Read the model definition and answer for the solid it produces. Units are mm, in the model's axes. Face numbers are marked on the shaded views. A direction names the side the tool comes from. Round coordinates to 2 decimals unless told otherwise and drop trailing zeros. Write each loop counter-clockwise with the first axis right and the second up, starting at its lowest first coordinate (ties: lowest second). Pieces come first, ordered by that corner, then holes. Notation, with made-up numbers: (8, 88) - (64, 88) arc R27 ccw to (64, 107) - close; hole circle Ø3 at (-29.75, -5). An arc over 180 degrees is marked (long way). Use one line per item in the form item = value. Start each with the question number.
1) Each of these flat-tipped pins is pushed along its axis until it touches: pin 1 (1.6 mm diameter, centred on x = 20.5, z = -1, fed in from +Y); pin 2 (3 mm diameter, centred on x = 15.41, z = -16.25, fed in from -Y); pin 3 (1.1 mm diameter, centred on x = 9, y = 3.5, fed in from -Z). Where does it stop, or does it pass through?
2) The part is cut by section B-B, the plane x = 21.75. Give the vertices of the cut face in (y, z), plus the area to 3 significant figures.
3) The part is cut by section C-C, the plane z = -6.25. Give the vertices of the cut face in (x, y), plus the area to 3 significant figures.
4) For the marked faces 1, 2 and 3, determine the directions among +Z, -Z, +X, -X, +Y, -Y from which every point of the face is accessible in a straight line to the end or side of a thin tool.
5) Consider line 1 along X through (y, z) = (2.3, -11.25); line 2 along Z through (x, y) = (16, 1.6); line 3 along Z through (x, y) = (16, 3.85). Determine where each line is inside the solid, lowest interval first. Write a range as from..to.
6) The part is cut by section D-D, the plane z = -9.5. Give the vertices of the cut face in (x, y), plus the area to 3 significant figures.
7) The part is cut by section A-A, the plane y = 3.35. Give the vertices of the cut face in (x, z).
from build123d import *

# Parameters (mm, degrees)
SKETCH_1_R          = 1.05
EXTRUDE_1_DEPTH     = 2
EXTRUDE_START       = 2
SKETCH_1_3_R        = 1.05
EXTRUDE_2_DEPTH     = 2.25
CUT_EXTRUDE_1_DEPTH = 2
SKETCH_3_R          = 1.15
CUT_EXTRUDE_2_DEPTH = 5.25
CHAMFER_1_SIZE      = 1.2


with BuildPart() as part:
    # Эскиз1 → Бобышка-Вытянуть1 (new body)
    with BuildSketch(Plane(origin=(0, 0, 0), x_dir=(1, 0, 0), z_dir=(0, 1, 0))):
        with BuildLine():
            Line((0.878934798, 22.5), (0.878934798, 20.5))
            ThreePointArc((0.878934798, 20.5), (2.615780546, 11.25), (0.878934798, 2))
            Line((0.878934798, 2), (0.878934798, 0))
            Line((0.878934798, 0), (27, 0))
            ThreePointArc((27, 0), (29.615780546, 11.25), (27, 22.5))
            Line((27, 22.5), (0.878934798, 22.5))
        make_face()
        with Locations((16, 11.25)):
            Circle(SKETCH_1_R, mode=Mode.SUBTRACT)
    extrude(amount=EXTRUDE_1_DEPTH)

    # Эскиз1<3> → Бобышка-Вытянуть2 (add)
    with BuildSketch(Plane(origin=(0, 0, 0), x_dir=(1, 0, 0), z_dir=(0, 1, 0)).offset(EXTRUDE_START)):
        with BuildLine():
            Line((27.878934798, 20.5), (0.878934798, 20.5))
            ThreePointArc((0.878934798, 20.5), (2.615780546, 11.25), (0.878934798, 2))
            Line((0.878934798, 2), (27.878934798, 2))
            ThreePointArc((27.878934798, 2), (29.615780546, 11.25), (27.878934798, 20.5))
        make_face()
        with Locations((16, 11.25)):
            Circle(SKETCH_1_3_R, mode=Mode.SUBTRACT)
    extrude(amount=EXTRUDE_2_DEPTH)

    # Эскиз2 → Вырез-Вытянуть1 (cut)
    with BuildSketch(Plane.XZ):
        with BuildLine():
            Line((6.079834852, 0), (0.878934798, 0))
            Line((0.878934798, 0), (0.878934798, -22.5))
            Line((0.878934798, -22.5), (6.079834852, -22.5))
            ThreePointArc((6.079834852, -22.5), (2.615780546, -11.25), (6.079834852, 0))
        make_face()
    extrude(amount=-CUT_EXTRUDE_1_DEPTH, mode=Mode.SUBTRACT)

    # Эскиз3 → Вырез-Вытянуть2 (cut, through all)
    with BuildSketch(Plane(origin=(0, 4.25, 0), x_dir=(1, 0, 0), z_dir=(0, 1, 0))):
        with Locations((15.410523666, 6.25)):
            Circle(SKETCH_3_R)
        with Locations((15.410523666, 16.25)):
            Circle(SKETCH_3_R)
    extrude(amount=-CUT_EXTRUDE_2_DEPTH, mode=Mode.SUBTRACT)

    # Фаска1
    chamfer_1_edges = [part.edges().sort_by_distance(p)[0] for p in [
        (14.260523666, 0, -16.25),
        (14.260523666, 0, -6.25),
    ]]
    chamfer(chamfer_1_edges, length=CHAMFER_1_SIZE)


solid = part.part
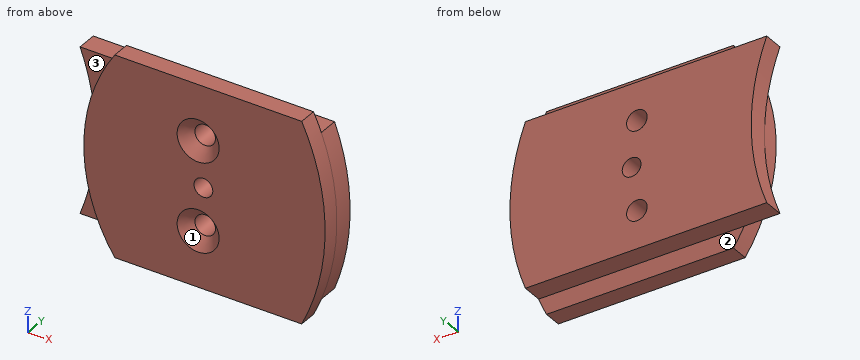
Geometry results:
q1.pin_1 = 2
q1.pin_2 = 0.85
q1.pin_3 = -20.5
q2.outline = (0, -22.5) - (2, -22.5) - (2, -20.5) - (4.25, -20.5) - (4.25, -2) - (2, -2) - (2, 0) - (0, 0) - close
q2.area = 86.6 mm2
q3.outline = (2.12, 2) - (3.25, 2) - (3.25, 0) - (13.06, 0) - (14.26, 1.2) - (14.26, 4.25) - (2.12, 4.25) - close; (16.56, 1.2) - (17.76, 0) - (29.12, 0) - (29.12, 4.25) - (16.56, 4.25) - close
q3.area = 101 mm2
q4.face_1 = -Y
q4.face_2 = -Z, +X, -X, +Y
q4.face_3 = +Z, -X, -Y
q5.line_1 = 2.62..14.95, 17.05..29.62
q5.line_2 = -22.5..-17.24, -15.26..-12.3, -10.2..-7.24, -5.26..0
q5.line_3 = -20.5..-17.24, -15.26..-12.3, -10.2..-7.24, -5.26..-2
q6.outline = (2.56, 2) - (2.69, 2) - (2.69, 0) - (29.56, 0) - (29.56, 4.25) - (2.56, 4.25) - close
q6.area = 114 mm2
q7.outline = (0.88, -20.5) - (27.88, -20.5) arc R25.5 ccw to (27.88, -2) - (0.88, -2) arc R25.5 cw to start; hole circle Ø2.3 at (15.41, -16.25); hole circle Ø2.3 at (15.41, -6.25); hole circle Ø2.1 at (16, -11.25)
